Design review of the part shown in the three views and the two pictorial views. Dimensions are in mm from the part's minimum x, y and z. A direction names the side the tool comes from. Coordinates: 2 decimals unless noted, no trailing zeros. Loops run counter-clockwise (first coordinate to the right, second up) from the corner with the lowest first, then second, coordinate; pieces in that order, holes last.
Q1. Add section B-B on z = 540. Give the boundary of the cut face in (x, y), and give its area (3 significant figures).
Q2. Add section A-A on x = 82.5. Give the boundary of the cut face in (y, z).
Q3. Machinability: for the marked faces 1 and 2, which of the approach directions +Z, -Z, +X, -X, +Y, -Y give a long, thin tool a straight path to every point of the face, cutting with its end or side? Answer none if there is none.
Q4. Add section C-C on y = 82.5. Give the boundary of the cut face in (x, z), and give its area (3 significant figures).
Q5. Wall thickness on probe 1 along X at (y, z) = (88.5, 153); probe 2 along Y at (x, z) = (70.5, 421); probe 3 along X at (y, z) = (155, 92.5): over which ranges is each line inside the solid? List them lowest first.
Q6. For P1, Ø3, axis at x = 159.5, y = 101, coming from the +Z side; P2, Ø1.5, axis at x = 339.5, y = 100.5, coming from the +Z side; P3, Ø4, axis at y = 101, z = 104.5, coming from the -X side, all flat-tipped, find the tip position at first contact; note any pin that passes through.
Q7. Draft analysis for pull direction Y (two halves, no side actions). For the marked faces 3, 4 and 5, state which applies: released by +Y, released by -Y, zero draft, split by the parting line, or undercut.
Q8. Add section D-D on y = 148. Give the boundary of the cut face in (x, z), and give its area (3 significant figures).
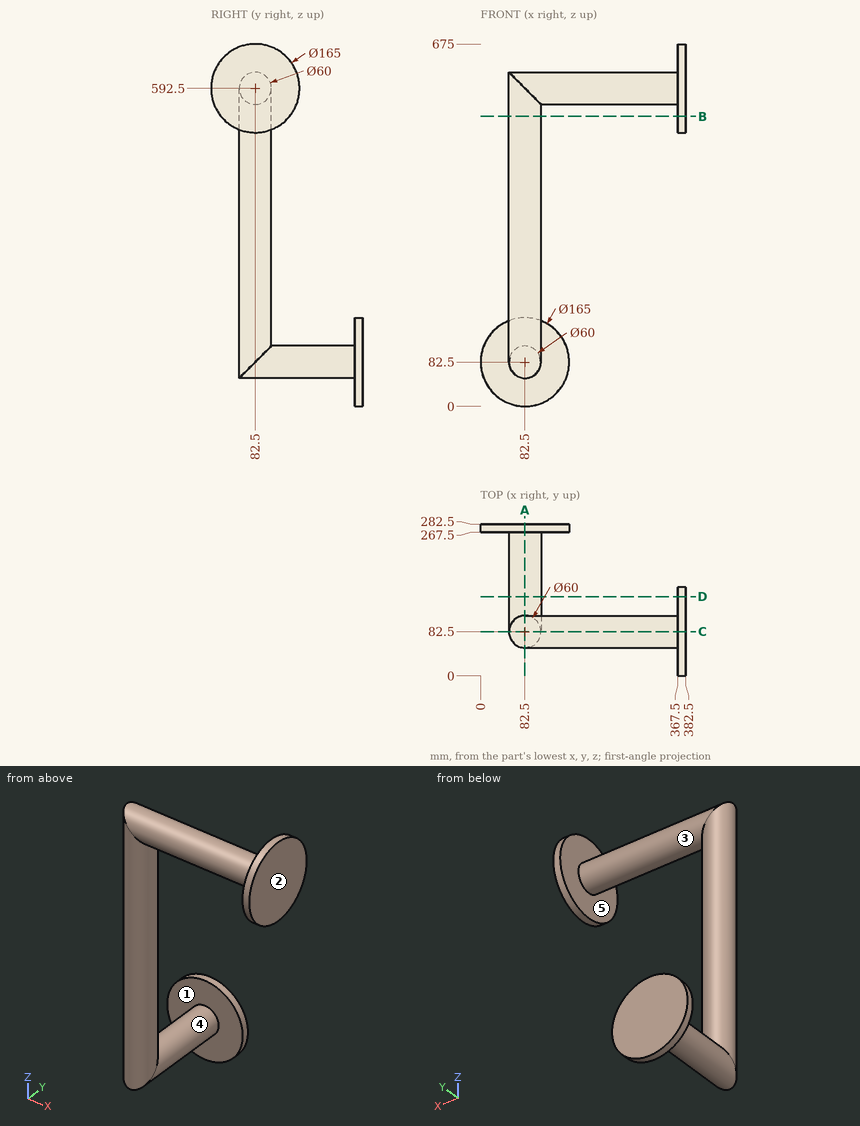
Entries:
1. outline: circle Ø60 at (82.5, 82.5); (367.5, 18.86) - (382.5, 18.86) - (382.5, 146.14) - (367.5, 146.14) - close
1. area: 4,740 mm2
2. outline: (52.5, 52.5) - (267.5, 52.5) - (267.5, 0) - (282.5, 0) - (282.5, 165) - (267.5, 165) - (267.5, 112.5) - (112.5, 112.5) - (112.5, 592.5) arc R30 ccw to (52.5, 592.5) - close
3. face 1: none
3. face 2: +Z, -Z, +X, +Y, -Y
4. outline: (52.5, 82.5) arc R30 ccw to (112.5, 82.5) - (112.5, 562.5) - (367.5, 562.5) - (367.5, 510) - (382.5, 510) - (382.5, 675) - (367.5, 675) - (367.5, 622.5) - (52.5, 622.5) - close
4. area: 51,600 mm2
5. probe 1: x = 53.11 to 111.89
5. probe 2: y = 55 to 110
5. probe 3: x = 54.22 to 110.78
6. P1: stops at z = 617.22
6. P2: stops at z = 617.04
6. P3: stops at x = 57.45
7. face 3: split by the parting line
7. face 4: undercut
7. face 5: zero draft
8. outline: circle Ø60 at (82.5, 82.5); (367.5, 542.34) - (382.5, 542.34) - (382.5, 642.66) - (367.5, 642.66) - close
8. area: 4,330 mm2
